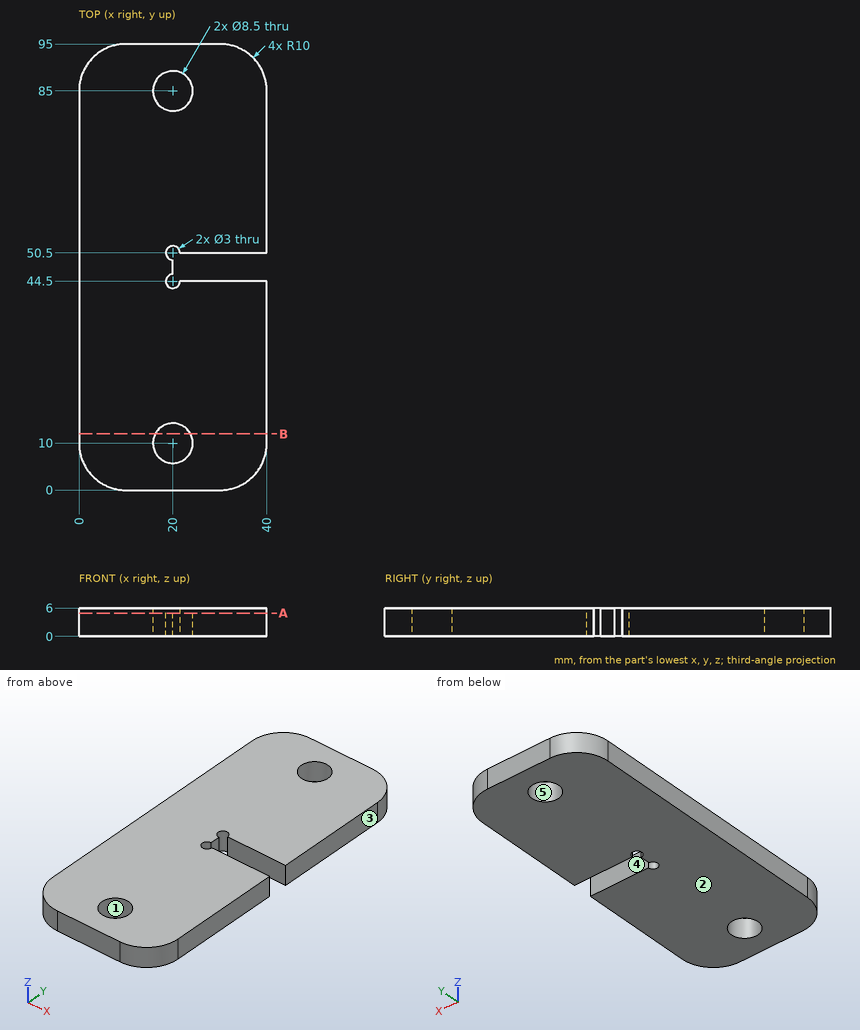
For this review, use the dimensioned drawing (mm, ordinates from the lowest corner) and the shaded views. A direction names the side the tool comes from. Round coordinates to 2 decimals unless told otherwise and drop trailing zeros. Order: outer loops, then holes, each group sorted by start corner. A loop starts at its lowest first (then second) coordinate and runs counter-clockwise, first axis right, second up. Notation, with made-up numbers: M 9,-4 L 19,-4 A20 ccw 19,32 Z; hole C 14.25,4.5 d3. An arc over 180 degrees is marked long. Write each question's results on one line, items separated by ' | '. Start each with the question number.
1. To check wall thickness, follow L1, parallel to Y at x = 17, z = 2.9; L2, parallel to Y at x = 26, z = 1.15; L3, parallel to Y at x = 37, z = 2. State the ranges of each line that lie inside material, in increasing order. Write a range as [from, to].
2. Clearance check with flat-ended pins moving along their axes: pin 1 Ø2.5 at (y, z) = (48, 2.5) entering from +X; pin 2 Ø2.5 at (x, y) = (20, 44.5) entering from +Z. State where each tip first meets the part, or that it passes through.
3. Tool access review of the marked faces 4 and 5: name each direction out of +Z, -Z, +X, -X, +Y, -Y from which nothing blocks a thin tool from reaching the whole face with its end or side.
4. Add section B-B (y = 12). State the section outline as (x, z) points, then the cut area to 3 significant figures.
5. Draft analysis for pull direction X (two halves, no side actions). For the marked faces 1, 2 and 3, state which applies: pulls with the +X half, pulls with the -X half, needs draft (parallel to the pull), parting line crosses it, or undercut.
6. Add section A-A (z = 4.95). State the section outline as (x, y) points, then the cut area to 3 significant figures.
Output values:
1) L1: [0, 6.99], [13.01, 81.99], [88.01, 95] | L2: [0, 44.5], [50.5, 95] | L3: [2.86, 44.5], [50.5, 92.14]
2) pin 1: x = 20 | pin 2: through
3) face 4: +Z, -Z, +X | face 5: +Z, -Z
4) outline: M 0,0 L 16.25,0 L 16.25,6 L 0,6 Z; M 23.75,0 L 40,0 L 40,6 L 23.75,6 Z | area: 195 mm^2
5) face 1: undercut | face 2: needs draft | face 3: pulls with the +X half
6) outline: M 0,10 A10 ccw 10,0 L 30,0 A10 ccw 40,10 L 40,44.5 L 21.5,44.5 A1.5 cw long 20,46 L 20,49 A1.5 cw long 21.5,50.5 L 40,50.5 L 40,85 A10 ccw 30,95 L 10,95 A10 ccw 0,85 Z; hole C 20,10 d8.5; hole C 20,85 d8.5 | area: 3,470 mm^2
